Read the model definition and answer for the solid it produces. Units are mm, in the model's axes. Face numbers are marked on the shaded views. A direction names the side the tool comes from. Coordinates: 2 decimals unless noted, no trailing zeros. Loops run counter-clockwise (first coordinate to the right, second up) from the corner with the lowest first, then second, coordinate; pieces in that order, holes last. Notation, with made-up numbers: (87, 85.25) -> (130, 85.25) arc R17 ccw to (130, 117.25) -> close; hole circle Ø10 at (42.25, -20.75). An arc over 180 degrees is marked (long way). Answer as a JSON object with one key per item and string values. Group by question number.
Q1. The part is cut by section A-A on x = -17. Write down the section's boundary in (y, z).
Q2. For the marked faces 1, 2 and 3, determine the directions among +Z, -Z, +X, -X, +Y, -Y from which every point of the face is accessible in a straight line to the end or side of a thin tool.
Q3. The part is cut by section C-C on x = 6.5. Write down the section's boundary in (y, z).
Q4. Straight lines are drawn through the part: line 1 along X through (y, z) = (1.7, -5.5); line 2 along Y through (x, z) = (-8.5, -7); line 3 along Z through (x, y) = (-13.5, 0.05). For each, find the intervals that lie inside material, in ascending order. Write a range as [from, to].
Q5. Each of these flat-tipped pins is pushed along its axis until it touches: P1, Ø0.6, axis at y = 0.5, z = 2.5, coming from the -X side; P2, Ø1, axis at x = -1, y = 0.5, coming from the -Z side; P3, Ø2.5, axis at x = 7, y = -2, coming from the +Z side; P4, Ø10, axis at x = 1.5, z = -5.5, coming from the -Y side. Where does it stop, or does it pass through?
Q6. The part is cut by section D-D on y = 1.5. Write down the section's boundary in (x, z), and give its area (4 significant figures).
Q7. The part is cut by section B-B on z = -5.5. Write down the section's boundary in (x, y).
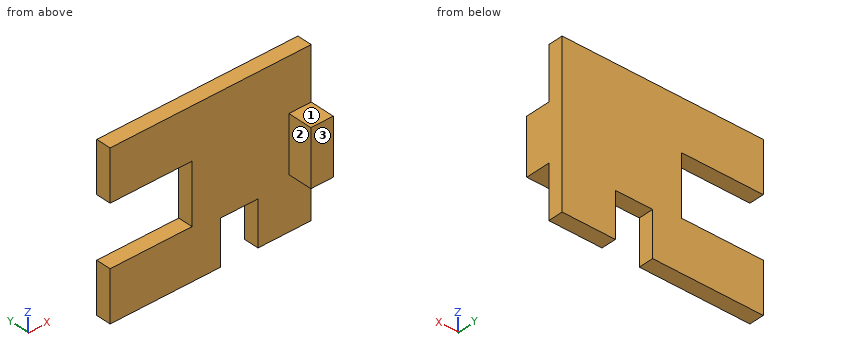
from build123d import *

# Parameters (mm, degrees)
BOSS_EXTRUDE1_DEPTH = 2
SKETCH2_W           = 3
SKETCH2_H           = 7.46
BOSS_EXTRUDE2_DEPTH = 3.3


with BuildPart() as part:
    # Sketch1 → Boss-Extrude1 (new body)
    with BuildSketch(Plane(origin=(0, 0, 0), x_dir=(1, 0, 0), z_dir=(0, 1, 0))):
        Polygon((-19.033651007, 9.961336175), (-4.183651007, 9.961336175), (-4.183651007, 3.961336175), (0.816348993, 3.961336175), (0.816348993, 9.961336175), (7.966348993, 9.961336175), (7.966348993, -11.538663825), (-19.033651007, -11.538663825), (-19.033651007, -4.788663825), (-8.033651007, -4.788663825), (-8.033651007, 3.211336175), (-19.033651007, 3.211336175), align=None)
    extrude(amount=BOSS_EXTRUDE1_DEPTH)

    # Sketch2 → Boss-Extrude2 (add)
    with BuildSketch(Plane.XZ):
        with Locations((6.466348993, 0.788663825)):
            Rectangle(SKETCH2_W, SKETCH2_H)
    extrude(amount=BOSS_EXTRUDE2_DEPTH)


solid = part.part
Final values:
{
 "1": {"outline": "(0, -9.96) -> (2, -9.96) -> (2, -3.21) -> (0, -3.21) -> close; (0, 4.79) -> (2, 4.79) -> (2, 11.54) -> (0, 11.54) -> close"},
 "2": {"face 1": "+Z, +X, -X, -Y", "face 2": "+Z, -Z, -X, -Y", "face 3": "+Z, -Z, +X, -X, -Y"},
 "3": {"outline": "(-3.3, -2.94) -> (0, -2.94) -> (0, -9.96) -> (2, -9.96) -> (2, 11.54) -> (0, 11.54) -> (0, 4.52) -> (-3.3, 4.52) -> close"},
 "4": {"line 1": "x = [-19.03, -4.18], [0.82, 7.97]", "line 2": "y = [0, 2]", "line 3": "z = [-9.96, -3.21], [4.79, 11.54]"},
 "5": {"P1": "stops at x = -8.03", "P2": "stops at z = -3.96", "P3": "stops at z = 4.52", "P4": "stops at y = -3.3"},
 "6": {"outline": "(-19.03, -9.96) -> (-4.18, -9.96) -> (-4.18, -3.96) -> (0.82, -3.96) -> (0.82, -9.96) -> (7.97, -9.96) -> (7.97, 11.54) -> (-19.03, 11.54) -> (-19.03, 4.79) -> (-8.03, 4.79) -> (-8.03, -3.21) -> (-19.03, -3.21) -> close", "area": "462.5 mm2"},
 "7": {"outline": "(-19.03, 0) -> (-4.18, 0) -> (-4.18, 2) -> (-19.03, 2) -> close; (0.82, 0) -> (7.97, 0) -> (7.97, 2) -> (0.82, 2) -> close"}
}
